Read the model definition and answer for the solid it produces. Units are mm, in the model's axes. Face numbers are marked on the shaded views. A direction names the side the tool comes from. Coordinates: 2 decimals unless noted, no trailing zeros. Write each loop counter-clockwise with the first axis right and the second up, starting at its lowest first coordinate (ties: lowest second). Pieces come first, ordered by that corner, then holes. Notation, with made-up numbers: (11.5, 59) - (56.5, 59) arc R7 ccw to (56.5, 72) - close; hole circle Ø1 at (34, 78). An arc over 180 degrees is marked (long way). Return JSON: item names as keys, results as strings.
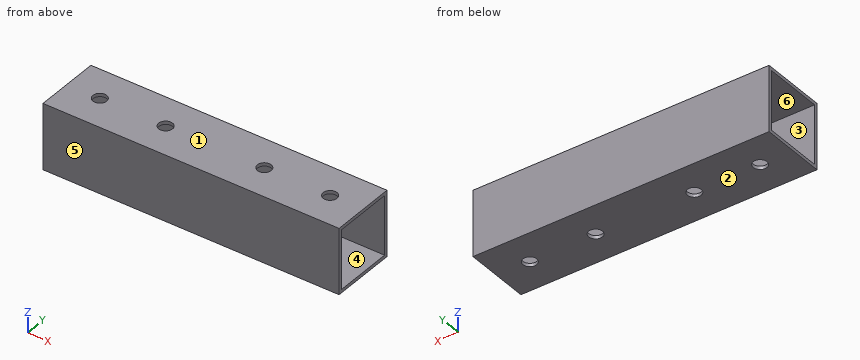
```python
from build123d import *

# Parameters (mm, degrees)
SKETCH_1_W          = 20
SKETCH_1_H          = 20
EXTRUDE_1_DEPTH     = 90
SKETCH_2_R          = 2.1
CUT_EXTRUDE_1_DEPTH = 93.736184955
SKETCH_3_W          = 18
SKETCH_3_H          = 18
CUT_EXTRUDE_2_DEPTH = 92.104335791


with BuildPart() as part:
    # 草图1 → 凸台-拉伸1 (new body)
    with BuildSketch(Plane(origin=(0, 0, 0), x_dir=(0, 0, -1), z_dir=(1, 0, 0))):
        Rectangle(SKETCH_1_W, SKETCH_1_H)
    extrude(amount=EXTRUDE_1_DEPTH)

    # 草图2 → 切除-拉伸1 (cut, through all)
    with BuildSketch(Plane.XY.offset(10)):
        with Locations((10, 0)):
            Circle(SKETCH_2_R)
        with Locations((30, 0)):
            Circle(SKETCH_2_R)
        with Locations(Location((60, 0, 0), (0, 0, 180))):
            Circle(SKETCH_2_R)
        with Locations(Location((80, 0, 0), (0, 0, 180))):
            Circle(SKETCH_2_R)
    extrude(amount=-CUT_EXTRUDE_1_DEPTH, mode=Mode.SUBTRACT)

    # 草图3 → 切除-拉伸2 (cut, through all)
    with BuildSketch(Plane.ZY):
        Rectangle(SKETCH_3_W, SKETCH_3_H)
    extrude(amount=-CUT_EXTRUDE_2_DEPTH, mode=Mode.SUBTRACT)


solid = part.part
```
(1) A cutting plane is placed at B-B (x = 48.5). Determine the outline of the cut face in (y, z).
Answer:
{"outline": "(-10, -10) - (10, -10) - (10, 10) - (-10, 10) - close; hole (-9, -9) - (9, -9) - (9, 9) - (-9, 9) - close"}
(2) Which of the six approach directions +Z, -Z, +X, -X, +Y, -Y give full straight-line access (tool end or side, diameter ignored) to the marked faces 5 and 6?
Answer:
{"face 5": "+Z, -Z, +X, -X, -Y", "face 6": "+X, -X"}
(3) Determine the mould class of the marked faces 1, 2, 3 and 4 for opening direction Z: +Z half, -Z half, draft (parallel to the pull), parting line (faces both ways), or undercut.
Answer:
{"face 1": "+Z half", "face 2": "-Z half", "face 3": "undercut", "face 4": "undercut"}
(4) A cutting plane is placed at A-A (z = 4). Determine the outline of the cut face in (x, y), and give its area (3 significant figures).
Answer:
{"outline": "(0, -10) - (90, -10) - (90, -9) - (0, -9) - close; (0, 9) - (90, 9) - (90, 10) - (0, 10) - close", "area": "180 mm²"}
(5) A cutting plane is placed at D-D (x = 80). Determine the outline of the cut face in (y, z).
Answer:
{"outline": "(-10, -10) - (-2.1, -10) - (-2.1, -9) - (-9, -9) - (-9, 9) - (-2.1, 9) - (-2.1, 10) - (-10, 10) - close; (2.1, -10) - (10, -10) - (10, 10) - (2.1, 10) - (2.1, 9) - (9, 9) - (9, -9) - (2.1, -9) - close"}
(6) Flat-ended cylindrical pins translate along their axes: P1, Ø3.5, axis at x = 80, y = 0, coming from the +Z side; P2, Ø5.5, axis at x = 10, y = 0, coming from the -Z side. Find the tip coordinate at first contact, or state that the pin passes through.
Answer:
{"P1": "through", "P2": "z = -10"}
(7) Straight lines are drawn through the part: line 1 (Y direction, x = 16, z = 2); line 2 (Y direction, x = 80, z = 9.2). For each, find the intervals that lie inside material, in ascending order. Write a range as from..to.
Answer:
{"line 1": "-10..-9, 9..10", "line 2": "-10..-2.1, 2.1..10"}
